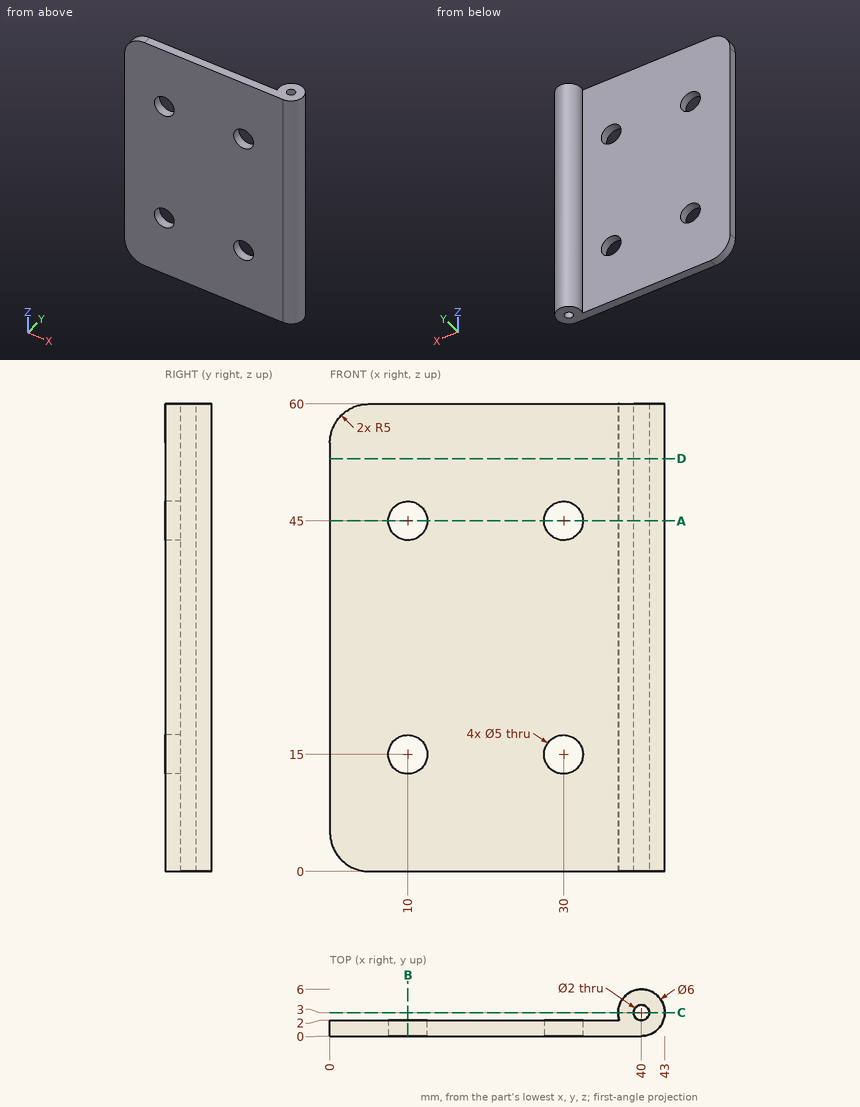
The figure shows three views and two pictorial views of one solid part (mm, origin at its lowest corner). Answer the questions. Coordinates: 2 decimals unless noted, no trailing zeros. Loops run counter-clockwise (first coordinate to the right, second up) from the corner with the lowest first, then second, coordinate; pieces in that order, holes last. Notation, with made-up numbers: (56.5, -14) -> (98.5, -14) arc R31 ccw to (98.5, 23) -> close; hole circle Ø5 at (-26, 9). An arc over 180 degrees is marked (long way). Write item = value, one per line. Start each with the question number.
1) A cutting plane is placed at B-B (x = 10). Give the vertices of the cut face in (y, z), then the cut area to 3 significant figures.
2) A cutting plane is placed at C-C (y = 3). Give the vertices of the cut face in (x, z).
3) Straight lines are drawn through the part: line 1 (Z direction, x = 10, y = 1); line 2 (Y direction, x = 40, z = 21); line 3 (X direction, y = 3, z = 43). For each, find the intervals that lie inside material, in ascending order. Write a range as from..to.
4) Given pin 1 Ø1 at (y, z) = (2, 41.5) entering from +X; pin 2 Ø6.5 at (x, z) = (10, 15) entering from +Y; pin 3 Ø2 at (y, z) = (1, 18.5) entering from +X, each flat-ended and moving along its own axis, determine where each tip first touches the part or whether it passes through.
5) A cutting plane is placed at D-D (z = 53). Give the vertices of the cut face in (x, y), then the cut area to 3 significant figures.
6) A cutting plane is placed at A-A (z = 45). Give the vertices of the cut face in (x, y).
Responses:
q1.outline = (0, 0) -> (2, 0) -> (2, 12.5) -> (0, 12.5) -> close; (0, 17.5) -> (2, 17.5) -> (2, 42.5) -> (0, 42.5) -> close; (0, 47.5) -> (2, 47.5) -> (2, 60) -> (0, 60) -> close
q1.area = 100 mm²
q2.outline = (37, 0) -> (39, 0) -> (39, 60) -> (37, 60) -> close; (41, 0) -> (43, 0) -> (43, 60) -> (41, 60) -> close
q3.line_1 = 0..12.5, 17.5..42.5, 47.5..60
q3.line_2 = 0..2, 4..6
q3.line_3 = 37..39, 41..43
q4.pin_1 = 42.96
q4.pin_2 = 2
q4.pin_3 = 42.83
q5.outline = (0, 0) -> (40, 0) arc R3 ccw (long way) to (37.17, 2) -> (0, 2) -> close; hole circle Ø2 at (40, 3)
q5.area = 101 mm²
q6.outline = (0, 0) -> (7.5, 0) -> (7.5, 2) -> (0, 2) -> close; (12.5, 0) -> (27.5, 0) -> (27.5, 2) -> (12.5, 2) -> close; (32.5, 0) -> (40, 0) arc R3 ccw (long way) to (37.17, 2) -> (32.5, 2) -> close; hole circle Ø2 at (40, 3)
